Design review of the part built by this model. Coordinates are the model's own, in mm. A direction names the side the tool comes from. Give positions to 0.01 mm unless a question says otherwise; leave off trailing zeros. Order: outer loops, then holes, each group sorted by start corner. A loop starts at its lowest first (then second) coordinate and runs counter-clockwise, first axis right, second up. Notation, with made-up numbers: (25.5, 31.25) -> (65.5, 31.25) arc R14 ccw to (65.5, 38.25) -> close; hole circle Ø5 at (84.5, -18.5). An arc over 180 degrees is marked (long way). Answer in a Markdown table with one row per item. Add a question column.
Autodesk Inventor part; units mm, degrees
ref_plane "YZ Plane" through (0, 0, 0) normal (1, 0, 0) x (0, 1, 0)
ref_plane "XZ Plane" through (0, 0, 0) normal (0, 1, 0) x (-1, 0, 0)
ref_plane "XY Plane" through (0, 0, 0) normal (0, 0, 1) x (1, 0, 0)
sketch "0" plane through (0, 0, 0) normal (0, 0, 1) x (1, 0, 0)
  line L0 (-44.5, -5) -> (-44.5, 5)
  line L1 (-44.5, 5) -> (-38.5, 5)
  line L2 (-38.5, 11) -> (-38.5, 9.5)
  line L3 (-38.5, 9.5) -> (-32.25, 9.5)
  line L4 (-23.5, 9.5) -> (-23.5, 6.5)
  line L5 (-23.5, 6.5) -> (-29.75, 6.5)
  line L6 (-32.25, 5.25) -> (-32.25, 6.5)
  line L7 (-32.25, 10.75) -> (-29.75, 10.75)
  line L8 (-29.75, 10.75) -> (-29.75, 9.5)
  line L9 (-29.75, 5.25) -> (-32.25, 5.25)
  line L10 (-32.25, 6.5) -> (-38.5, 6.5)
  line L11 (-29.75, 6.5) -> (-29.75, 5.25)
  line L12 (-32.25, 9.5) -> (-32.25, 10.75)
  line L13 (-38.5, 6.5) -> (-38.5, 5)
  line L14 (-44.5, 11) -> (-44.5, 21)
  line L15 (-38.5, 11) -> (-44.5, 11)
  line L16 (-44.5, 21) -> (-38.5, 21)
  line L17 (-29.75, 9.5) -> (-23.5, 9.5)
  line L18 (38.5, 21) -> (44.5, 21)
  line L19 (44.5, 21) -> (44.5, 11)
  line L20 (44.5, 11) -> (38.5, 11)
  line L21 (38.5, 5) -> (38.5, 6.5)
  line L22 (38.5, 6.5) -> (32.25, 6.5)
  line L23 (23.5, 6.5) -> (23.5, 9.5)
  line L24 (23.5, 9.5) -> (29.75, 9.5)
  line L25 (32.25, 10.75) -> (32.25, 9.5)
  line L26 (32.25, 5.25) -> (29.75, 5.25)
  line L27 (29.75, 5.25) -> (29.75, 6.5)
  line L28 (29.75, 10.75) -> (32.25, 10.75)
  line L29 (32.25, 9.5) -> (38.5, 9.5)
  line L30 (29.75, 9.5) -> (29.75, 10.75)
  line L31 (32.25, 6.5) -> (32.25, 5.25)
  line L32 (38.5, 9.5) -> (38.5, 11)
  line L33 (44.5, 5) -> (44.5, -5)
  line L34 (38.5, 5) -> (44.5, 5)
  line L35 (29.75, 6.5) -> (23.5, 6.5)
  line L36 (-38.5, 21) -> (38.5, 21)
  line L37 (38.5, -15) -> (13, -15)
  line L38 (13, -15) -> (13, -21)
  line L39 (-13, -21) -> (-13, -15)
  line L40 (-13, -15) -> (-38.5, -15)
  line L41 (-13, -21) -> (13, -21)
  line L42 (-44.5, -5) -> (-38.5, -5)
  line L43 (-38.5, -5) -> (-38.5, -15)
  line L44 (44.5, -5) -> (38.5, -5)
  line L45 (38.5, -5) -> (38.5, -15)
sketch "Эскиз3" plane through (0, 0, 0) normal (0, 0, 1) x (1, 0, 0)
  line L0 (-44.5, 21) -> (-38.5, 21)
  line L1 (-38.5, 21) -> (38.5, 21)
  line L2 (38.5, 21) -> (44.5, 21)
  line L3 (44.5, 21) -> (44.5, 11)
  line L4 (44.5, 11) -> (38.5, 11)
  line L5 (38.5, 5) -> (44.5, 5)
  line L6 (38.5, 5) -> (38.5, 6.5)
  line L7 (38.5, 9.5) -> (38.5, 11)
  line L8 (32.25, 9.5) -> (38.5, 9.5)
  line L9 (38.5, 6.5) -> (32.25, 6.5)
  line L10 (32.25, 6.5) -> (32.25, 5.25)
  line L11 (32.25, 5.25) -> (29.75, 5.25)
  line L12 (29.75, 5.25) -> (29.75, 6.5)
  line L13 (29.75, 10.75) -> (32.25, 10.75)
  line L14 (32.25, 10.75) -> (32.25, 9.5)
  line L15 (29.75, 9.5) -> (29.75, 10.75)
  line L16 (29.75, 6.5) -> (23.5, 6.5)
  line L17 (23.5, 9.5) -> (29.75, 9.5)
  line L18 (23.5, 6.5) -> (23.5, 9.5)
  line L19 (44.5, 5) -> (44.5, -5)
  line L20 (44.5, -5) -> (38.5, -5)
  line L21 (38.5, -5) -> (38.5, -15)
  line L22 (13, -15) -> (13, -21)
  line L23 (38.5, -15) -> (13, -15)
  line L24 (-13, -21) -> (13, -21)
  line L25 (-13, -21) -> (-13, -15)
  line L26 (-13, -15) -> (-38.5, -15)
  line L27 (-38.5, -5) -> (-38.5, -15)
  line L28 (-44.5, -5) -> (-38.5, -5)
  line L29 (-44.5, -5) -> (-44.5, 5)
  line L30 (-44.5, 5) -> (-38.5, 5)
  line L31 (-38.5, 6.5) -> (-38.5, 5)
  line L32 (-32.25, 6.5) -> (-38.5, 6.5)
  line L33 (-32.25, 5.25) -> (-32.25, 6.5)
  line L34 (-29.75, 5.25) -> (-32.25, 5.25)
  line L35 (-29.75, 6.5) -> (-29.75, 5.25)
  line L36 (-23.5, 6.5) -> (-29.75, 6.5)
  line L37 (-23.5, 9.5) -> (-23.5, 6.5)
  line L38 (-29.75, 9.5) -> (-23.5, 9.5)
  line L39 (-29.75, 10.75) -> (-29.75, 9.5)
  line L40 (-32.25, 10.75) -> (-29.75, 10.75)
  line L41 (-32.25, 9.5) -> (-32.25, 10.75)
  line L42 (-38.5, 9.5) -> (-32.25, 9.5)
  line L43 (-38.5, 11) -> (-38.5, 9.5)
  line L44 (-38.5, 11) -> (-44.5, 11)
  line L45 (-44.5, 11) -> (-44.5, 21)
  line L46 (-44.5, 21) -> (44.5, 21)
  line L47 (44.5, 21) -> (44.5, 11)
  line L48 (-44.5, 11) -> (-44.5, 21)
  line L49 (23.5, 6.5) -> (23.5, 9.5)
  line L50 (29.75, 10.75) -> (32.25, 10.75)
  line L51 (32.25, 5.25) -> (29.75, 5.25)
  line L52 (44.5, 5) -> (38.5, 5)
  line L53 (44.5, 5) -> (38.5, 5)
  line L54 (38.5, -5) -> (44.5, -5)
  line L55 (44.5, -5) -> (44.5, 5)
  line L56 (13, -15) -> (38.5, -15)
  line L57 (38.5, -15) -> (38.5, -5)
  line L58 (13, -21) -> (-13, -21)
  line L59 (-13, -21) -> (-13, -15)
  line L60 (13, -15) -> (13, -21)
  line L61 (-13, -15) -> (-38.5, -15)
  line L62 (-38.5, -15) -> (-38.5, -5)
  line L63 (-44.5, 5) -> (-38.5, 5)
  line L64 (-38.5, -5) -> (-44.5, -5)
  line L65 (-44.5, -5) -> (-44.5, 5)
  line L66 (-44.5, 5) -> (-38.5, 5)
  line L67 (-23.5, 9.5) -> (-23.5, 6.5)
  line L68 (-32.25, 10.75) -> (-29.75, 10.75)
  line L69 (-29.75, 5.25) -> (-32.25, 5.25)
  line L70 (-32.25, 5.25) -> (-32.25, 6.5)
  line L71 (-32.25, 9.5) -> (-32.25, 10.75)
  line L72 (-29.75, 10.75) -> (-29.75, 9.5)
  line L73 (-29.75, 6.5) -> (-29.75, 5.25)
  line L74 (-38.5, 9.5) -> (-32.25, 9.5)
  line L75 (-29.75, 9.5) -> (-23.5, 9.5)
  line L76 (-23.5, 6.5) -> (-29.75, 6.5)
  line L77 (-32.25, 6.5) -> (-38.5, 6.5)
  line L78 (29.75, 5.25) -> (29.75, 6.5)
  line L79 (29.75, 9.5) -> (29.75, 10.75)
  line L80 (32.25, 10.75) -> (32.25, 9.5)
  line L81 (32.25, 6.5) -> (32.25, 5.25)
  line L82 (23.5, 9.5) -> (29.75, 9.5)
  line L83 (32.25, 9.5) -> (38.5, 9.5)
  line L84 (38.5, 6.5) -> (32.25, 6.5)
  line L85 (29.75, 6.5) -> (23.5, 6.5)
  line L86 (38.5, 5) -> (38.5, 6.5)
  line L87 (38.5, 9.5) -> (38.5, 11)
  line L88 (-38.5, 5) -> (-38.5, 6.5)
  line L89 (-38.5, 9.5) -> (-38.5, 11)
  line L90 (44.5, 11) -> (38.5, 11)
  line L91 (-38.5, 11) -> (-44.5, 11)
  line L92 (-44.5, 11) -> (-44.5, 10.75)
  line L93 (-44.5, 5.25) -> (-44.5, 5)
  line L94 (44.5, 11) -> (44.5, 10.75)
  line L95 (44.5, 5.25) -> (44.5, 5)
  point P0 (0, 0)
extrude "Выдавливание2" add sketch "0" along normal blind 10
properties part number "Крепление_мотора3_платформа"
1) For L1, parallel to X at y = 5.5, z = 7.25; L2, parallel to Y at x = -25.5, z = 0.75; L3, parallel to X at y = -6.5, z = 2.25, list the stretches that pass through material, from the lowest coordinate up.
2) Mouldability with a two-part tool opening along X and no side actions: class faces 1 (the face through (31, 10.75, 5)), 2 (the face through (-44.5, 16, 5)), 3 (the face through (38.5, -10, 5)), 4 (the face through (42, -5, 5)) as +X half, -X half, draft (parallel to the pull), parting line (faces both ways), or undercut.
3) Add section A-A, the plane x = 27.5. Write out the cut boundary in (y, z).
4) Machinability: for faces 5 (the face through (35, 9.5, 5)), 6 (the face through (44.5, 0, 5)), 7 (the face through (13, -18, 5)), 8 (the face through (-13, -18, 5)), 9 (the face through (-23.5, 8, 5)), which of the approach directions +Z, -Z, +X, -X, +Y, -Y give a long, thin tool a straight path to every point of the face, cutting with its end or side? Answer none if there is none.
5) Clearance check with flat-ended pins moving along their axes: P1, Ø3, axis at x = 25.5, z = 3.5, coming from the -Y side; P2, Ø0.6, axis at y = 10, z = 6.5, coming from the +X side; P3, Ø2.5, axis at y = 7.5, z = 5, coming from the -X side. State where each tip first meets the part, or that it passes through.
Verdict:
| question | item | result |
|---|---|---|
| 1 | L1 | x = -38.5 to -32.25, -29.75 to 29.75, 32.25 to 38.5 |
| 1 | L2 | y = -15 to 6.5, 9.5 to 21 |
| 1 | L3 | x = -38.5 to 38.5 |
| 2 | face 1 | undercut |
| 2 | face 2 | -X half |
| 2 | face 3 | +X half |
| 2 | face 4 | draft |
| 3 | outline | (-15, 0) -> (6.5, 0) -> (6.5, 10) -> (-15, 10) -> close; (9.5, 0) -> (21, 0) -> (21, 10) -> (9.5, 10) -> close |
| 4 | face 5 | +Z, -Z, +X |
| 4 | face 6 | +Z, -Z, +X, +Y, -Y |
| 4 | face 7 | +Z, -Z, +X, -Y |
| 4 | face 8 | +Z, -Z, -X, -Y |
| 4 | face 9 | +Z, -Z, -X |
| 5 | P1 | stops at y = -15 |
| 5 | P2 | stops at x = 38.5 |
| 5 | P3 | stops at x = -38.5 |
